Study the drawing (mm; zero at the part's minimum x, y, z) and answer. Coordinates: 2 decimals unless noted, no trailing zeros. Order: outer loops, then holes, each group sorted by start corner. A loop starts at its lowest first (then second) coordinate and runs counter-clockwise, first axis right, second up. Notation, with made-up numbers: (47, -34) - (90, -34) arc R22 ccw to (90, 4) - close; hole circle Ø4 at (-20, 73). An arc over 180 degrees is marked (long way). Write item = value, one per line.
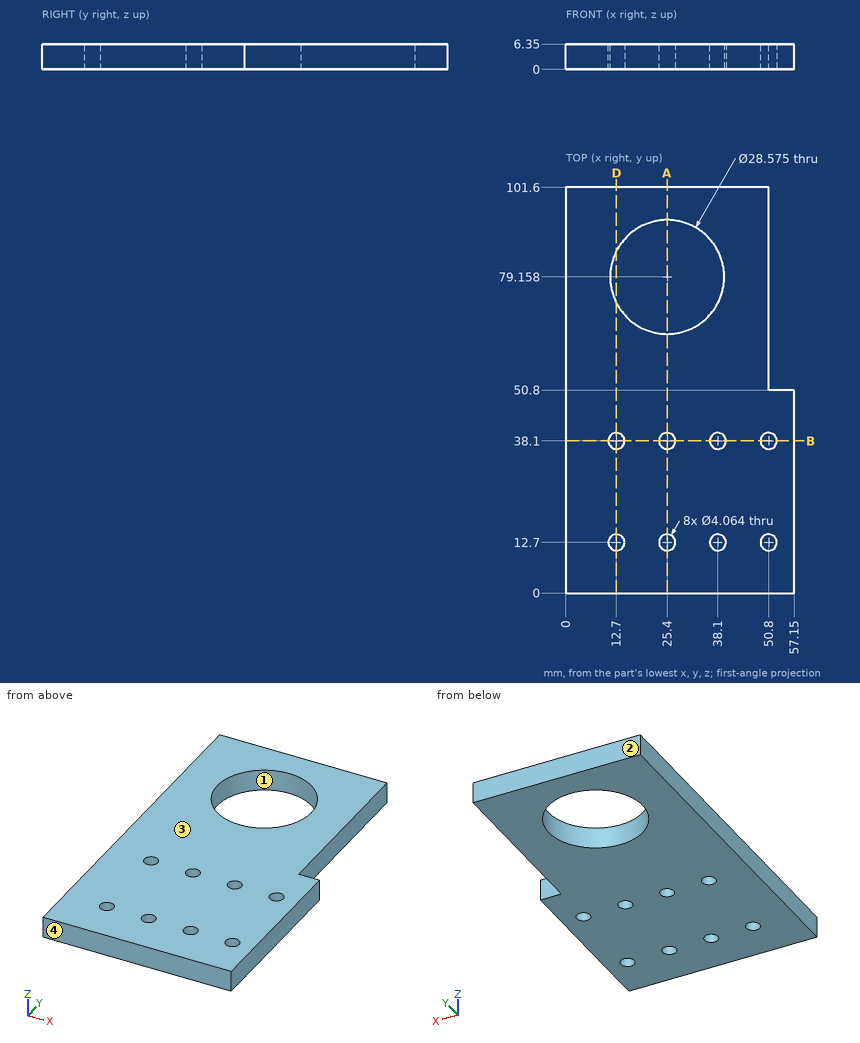
1) Straight lines are drawn through the part: line 1 along X through (y, z) = (12.7, 4.5); line 2 along Y through (x, z) = (25.4, 5) (1 decimal); line 3 along Y through (x, z) = (49, 5.5) (1 decimal). For each, find the intervals that lie inside material, in ascending order. Write a range as from..to.
Returned:
line_1 = 0..10.67, 14.73..23.37, 27.43..36.07, 40.13..48.77, 52.83..57.15
line_2 = 0..10.7, 14.7..36.1, 40.1..64.9, 93.4..101.6
line_3 = 0..11.8, 13.6..37.2, 39..101.6
2) The part is cut by section D-D (x = 12.7). Determine the outline of the cut face in (y, z).
Returned:
outline = (0, 0) - (10.67, 0) - (10.67, 6.35) - (0, 6.35) - close; (14.73, 0) - (36.07, 0) - (36.07, 6.35) - (14.73, 6.35) - close; (40.13, 0) - (72.61, 0) - (72.61, 6.35) - (40.13, 6.35) - close; (85.7, 0) - (101.6, 0) - (101.6, 6.35) - (85.7, 6.35) - close
3) The part is cut by section A-A (x = 25.4). Count the separate pieces of the cut face and the enclosed holes in it, and give its area (3 significant figures).
Returned:
separate_pieces = 4
enclosed_holes = 0
area = 412 mm^2
4) The part is cut by section B-B (y = 38.1). Determine the outline of the cut face in (x, z), and give its area (3 significant figures).
Returned:
outline = (0, 0) - (10.67, 0) - (10.67, 6.35) - (0, 6.35) - close; (14.73, 0) - (23.37, 0) - (23.37, 6.35) - (14.73, 6.35) - close; (27.43, 0) - (36.07, 0) - (36.07, 6.35) - (27.43, 6.35) - close; (40.13, 0) - (48.77, 0) - (48.77, 6.35) - (40.13, 6.35) - close; (52.83, 0) - (57.15, 0) - (57.15, 6.35) - (52.83, 6.35) - close
area = 260 mm^2
5) Flat-ended cylindrical pins translate along their axes: pin 1 Ø5 at (x, y) = (20, 56) entering from -Z; pin 2 Ø3 at (y, z) = (69, 4) entering from +X; pin 3 Ø17 at (x, y) = (25.4, 79.16) entering from +Z. Find the tip coordinate at first contact, or state that the pin passes through.
Returned:
pin_1 = 0
pin_2 = 50.8
pin_3 = through
6) Determine the mould class of the marked faces 1, 2, 3 and 4 for opening direction Y: pulls with the +Y half, pulls with the -Y half, needs draft (parallel to the pull), parting line crosses it, or undercut.
Returned:
face_1 = undercut
face_2 = pulls with the +Y half
face_3 = needs draft
face_4 = pulls with the -Y half
